from build123d import *

# Parameters (mm, degrees)
BOSS_EXTRUDE1_DEPTH = 4
BOSS_EXTRUDE2_DEPTH = 3
FILLET1_R           = 5
FILLET2_R           = 5


with BuildPart() as part:
    # Sketch1 → Boss-Extrude1 (new body)
    with BuildSketch(Plane.XY):
        with BuildLine():
            Line((-10.325, 10.325), (-10.325, -31.925))
            Line((-10.325, -31.925), (-18.1, -31.925))
            Line((-18.1, -31.925), (-18.1, -14.191194453))
            ThreePointArc((-18.1, -14.191194453), (0, 23), (18.1, -14.191194453))
            Line((18.1, -14.191194453), (18.1, -31.925))
            Line((18.1, -31.925), (10.325, -31.925))
            Line((10.325, -31.925), (10.325, 10.325))
            Line((10.325, 10.325), (10.325, 17.8))
            Line((10.325, 17.8), (-10.325, 17.8))
            Line((-10.325, 17.8), (-10.325, 10.325))
        make_face()
    extrude(amount=BOSS_EXTRUDE1_DEPTH)

    # Sketch2 → Boss-Extrude2 (add)
    with BuildSketch(Plane.XY.offset(4)):
        with BuildLine():
            Line((-10.325, -18.401205803), (-10.325, -20.55223528))
            ThreePointArc((-10.325, -20.55223528), (0, 23), (10.325, -20.55223528))
            Line((10.325, -20.55223528), (10.325, -18.401205803))
            ThreePointArc((10.325, -18.401205803), (0, 21.1), (-10.325, -18.401205803))
        make_face()
    extrude(amount=BOSS_EXTRUDE2_DEPTH)

    # Fillet1
    fillet1_edges = [part.edges().sort_by_distance(p)[0] for p in [
        (10.325, 17.8, 2),
        (-10.325, 17.8, 2),
    ]]
    fillet(fillet1_edges, radius=FILLET1_R)

    # Fillet2
    fillet2_edges = [part.edges().sort_by_distance(p)[0] for p in [
        (18.1, -31.925, 2),
        (-18.1, -31.925, 2),
        (-18.1, -14.191194453, 2),
        (18.1, -14.191194453, 2),
    ]]
    fillet(fillet2_edges, radius=FILLET2_R)


solid = part.part
Input: part model. Units: mm. Frame: model coordinates. A direction names the side the tool comes from. Give positions to 0.01 mm unless a question says otherwise; leave off trailing zeros. Order: outer loops, then holes, each group sorted by start corner. A loop starts at its lowest first (then second) coordinate and runs counter-clockwise, first axis right, second up.
Q1. Contact query for flat-ended pins moving along their axis: pin 1 Ø4.5 at (x, y) = (15.5, -27) entering from +Z; pin 2 Ø1.2 at (y, z) = (-19, 2) entering from -X; pin 3 Ø3 at (x, z) = (-2, 1.5) entering from -Y; pin 4 Ø10 at (x, y) = (-11, -20.5) entering from -Z. Output: stop coordinate, or through.
Checked values:
pin 1: stops at z = 4
pin 2: stops at x = -18.1
pin 3: stops at y = 17.8
pin 4: stops at z = 0
Q2. Section D-D on y = -25.5. Output: boundary loops of the cut face in (x, z) (3 decimals), and give its area (3 significant figures).
Checked values:
outline: (-18.1, 0) - (-10.325, 0) - (-10.325, 4) - (-18.1, 4) - close; (10.325, 0) - (18.1, 0) - (18.1, 4) - (10.325, 4) - close
area: 62.2 mm2
Q3. Section A-A on y = 0. Output: boundary loops of the cut face in (x, z) (3 decimals), and give its area (3 significant figures).
Checked values:
outline: (-23, 0) - (-10.325, 0) - (-10.325, 4) - (-21.1, 4) - (-21.1, 7) - (-23, 7) - close; (10.325, 0) - (23, 0) - (23, 7) - (21.1, 7) - (21.1, 4) - (10.325, 4) - close
area: 113 mm2
Q4. Section B-B on x = 0. Output: boundary loops of the cut face in (y, z), and give its area (3 significant figures).
Checked values:
outline: (17.8, 0) - (23, 0) - (23, 7) - (21.1, 7) - (21.1, 4) - (17.8, 4) - close
area: 26.5 mm2
Q5. Set-up query: faces 5 (the cylindrical face through (-8.899, 16.296, 2.028)), 6 (the flat face through (-15, -24, 4)), 7 (the flat face through (18.1, -21, 2)), 8 (the cylindrical face through (0.777, 21.086, 5.479)), 9 (the flat face through (15, -24, 4)). Return all of +Z, -Z, +X, -X, +Y, -Y with unobstructed straight access to the full face (end or side cutting, diameter ignored); none if empty.
Checked values:
face 5: +Z, -Z, -Y
face 6: +Z, -X, -Y
face 7: +Z, -Z, +X, -Y
face 8: +Z
face 9: +Z, +X, -Y
Q6. Draft query along X for faces 1 (the cylindrical face through (18.33, -14.32, 2.03)), 2 (the flat face through (-11, 3, 4)), 3 (the cylindrical face through (-16.596, -30.499, 2.028)), 4 (the flat face through (11, -4, 0)). Return one class per face: +X half, -X half, draft (parallel to the pull), parting line (faces both ways), or undercut.
Checked values:
face 1: +X half
face 2: undercut
face 3: -X half
face 4: draft
Q7. Section C-C on z = 3.25. Output: boundary loops of the cut face in (x, y) (3 decimals).
Checked values:
outline: (-18.975, -12.998) arc R5 cw to (-18.1, -15.824) - (-18.1, -26.925) arc R5 ccw to (-13.1, -31.925) - (-10.325, -31.925) - (-10.325, 12.8) arc R5 cw to (-5.325, 17.8) - (5.325, 17.8) arc R5 cw to (10.325, 12.8) - (10.325, -31.925) - (13.1, -31.925) arc R5 ccw to (18.1, -26.925) - (18.1, -15.824) arc R5 cw to (18.975, -12.998) arc R23 ccw (long way) to start
Q8. Ray query, probe 1 along X at (y, z) = (0, 5.5); probe 2 along X at (y, z) = (-20.5, 2.5) (3 decimals); probe 3 along Z at (x, y) = (14, -11.5). Return the intervals inside material, ascending.
Checked values:
probe 1: x = -23 to -21.1, 21.1 to 23
probe 2: x = -18.1 to -10.325, 10.325 to 18.1
probe 3: z = 0 to 4
